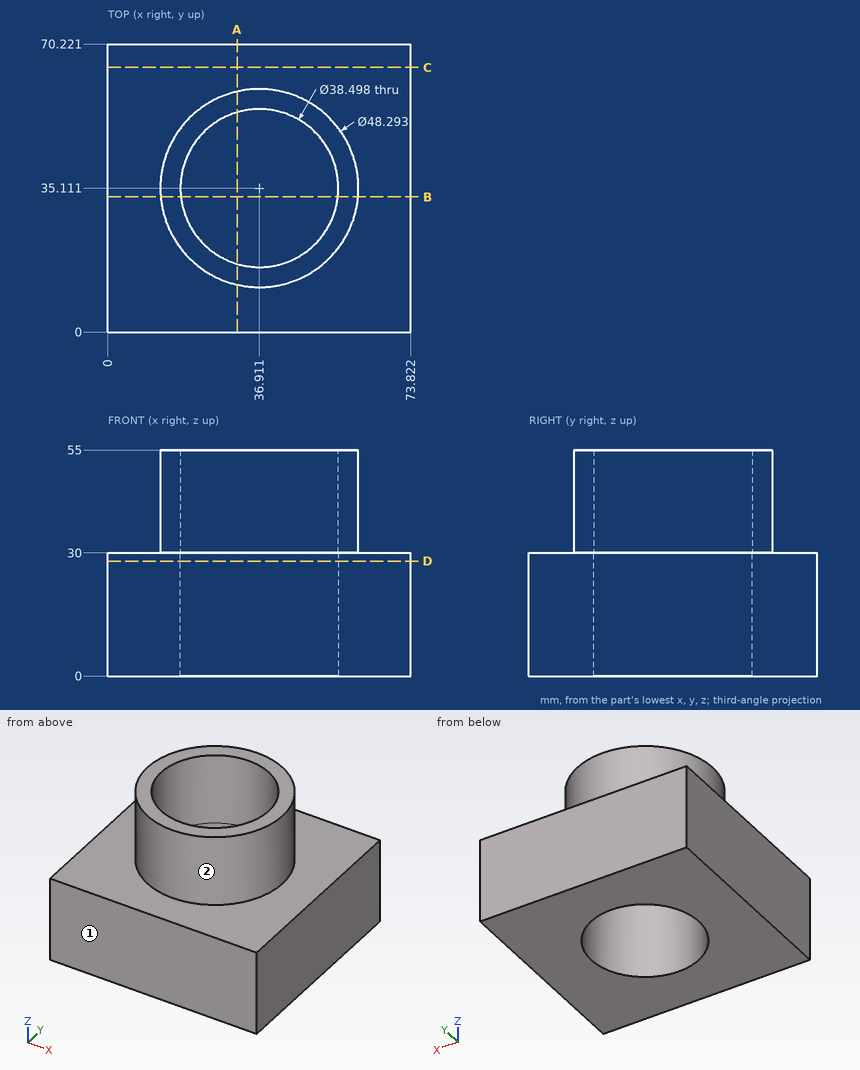
Design review of the part shown in the three views and the two pictorial views. Dimensions are in mm from the part's minimum x, y and z. A direction names the side the tool comes from. Give positions to 0.01 mm unless a question says otherwise; leave off trailing zeros. Loops run counter-clockwise (first coordinate to the right, second up) from the corner with the lowest first, then second, coordinate; pieces in that order, holes last. Notation, with made-up numbers: (-0.75, 69) - (29.25, 69) arc R25 ccw to (29.25, 92) - close; hole circle Ø7 at (20, 6.5). An arc over 180 degrees is marked (long way). Write item = value, one per line.
1) To check wall thickness, follow line 1 (X direction, y = 35, z = 52.5) (1 decimal); line 2 (X direction, y = 34.5, z = 19); line 3 (Z direction, x = 55.5, y = 17.5). State the ranges of each line that lie inside material, in increasing order.
Result sheet:
line_1 = 12.8 to 17.7, 56.2 to 61.1
line_2 = 0 to 17.67, 56.15 to 73.82
line_3 = 0 to 30
2) Clearance check with flat-ended pins moving along their axes: pin 1 Ø1.5 at (x, y) = (51.5, 11.5) entering from +Z; pin 2 Ø4 at (x, y) = (15.5, 40.5) entering from -Z; pin 3 Ø1 at (y, z) = (38, 43.5) entering from +X. State where each tip first meets the part, or that it passes through.
Result sheet:
pin_1 = 30
pin_2 = 0
pin_3 = 60.94
3) Tool access review of the marked faces 1 and 2: name each direction out of +Z, -Z, +X, -X, +Y, -Y from which nothing blocks a thin tool from reaching the whole face with its end or side.
Result sheet:
face_1 = +Z, -Z, +X, -X, -Y
face_2 = +Z
4) Take a section at B-B on y = 33. State the section outline as (x, z) points (1 decimal), and give its area (3 significant figures).
Result sheet:
outline = (0, 0) - (17.8, 0) - (17.8, 55) - (12.9, 55) - (12.9, 30) - (0, 30) - close; (56, 0) - (73.8, 0) - (73.8, 30) - (61, 30) - (61, 55) - (56, 55) - close
area = 1,310 mm2
5) Take a section at D-D on z = 28. State the section outline as (x, y) points.
Result sheet:
outline = (0, 0) - (73.82, 0) - (73.82, 70.22) - (0, 70.22) - close; hole circle Ø38.5 at (36.91, 35.11)
6) Take a section at A-A on x = 31.5. State the section outline as (y, z) points.
Result sheet:
outline = (0, 0) - (16.64, 0) - (16.64, 55) - (11.58, 55) - (11.58, 30) - (0, 30) - close; (53.58, 0) - (70.22, 0) - (70.22, 30) - (58.64, 30) - (58.64, 55) - (53.58, 55) - close
7) Take a section at C-C on y = 64.5. State the section outline as (x, z) points.
Result sheet:
outline = (0, 0) - (73.82, 0) - (73.82, 30) - (0, 30) - close
